The listing builds one solid part. Answer for the finished solid, in the listing's coordinates (mm). Face numbers are marked on the shaded views. Give positions to 0.01 mm unless a question says otherwise; leave off trailing zeros. Write each loop counter-clockwise with the first axis right and the second up, starting at its lowest first coordinate (ties: lowest second). Pieces come first, ordered by that corner, then holes. Notation, with made-up numbers: (-10.75, -6.75) - (24.25, -6.75) arc R5 ccw to (24.25, -1.75) - close; hole circle Ø5 at (-33.75, -27.5). An arc over 180 degrees is marked (long way). Answer as CSV lines item,"result". Start each with the question number.
(1) For a pull along Z with two mould halves and no side action, classify the marked faces 1, 2 and 3 as pulls with the +Z half, pulls with the -Z half, needs draft (parallel to the pull), parting line crosses it, or undercut.
(2) Find section C-C (x = 24.5). Write down the section's boundary in (y, z).
(3) Find section B-B (z = 14.5). Write down the section's boundary in (x, y).
(4) Straight lines are drawn through the part: probe 1 along X at (y, z) = (0.25, -11); probe 2 along Z at (x, y) = (-10.5, -2.75); probe 3 along X at (y, z) = (-13.25, 25). For each, find the intervals that lie inside material, in ascending order.
(5) Find section A-A (y = -1.75). State how many separate pieces and enclosed holes the cut face has, then the cut area to 3 significant figures.
(6) Each of these flat-tipped pins is pushed along its axis until it touches: pin 1 Ø0.8 at (y, z) = (1, -29.5) entering from +X; pin 2 Ø5 at (x, y) = (27, -3.5) entering from +Z; pin 3 Ø2.5 at (x, z) = (38.38, -39.22) entering from -Y; pin 4 Ø8 at (x, z) = (8.5, 22) entering from -Y. Where does it stop, or does it pass through?
from build123d import *

# Parameters (mm, degrees)
SKETCH1_R           = 1.375
BOSS_EXTRUDE1_DEPTH = 1.6
BOSS_EXTRUDE2_START = -17
BOSS_EXTRUDE2_DEPTH = 17
BOSS_EXTRUDE3_START = -17.6
SKETCH2_R           = 2.4
SKETCH2_R_2         = 1.375
BOSS_EXTRUDE3_DEPTH = 17.6
SKETCH3_W           = 36.288172123
SKETCH3_H           = 9.00941151
CUT_EXTRUDE1_DEPTH  = 10
SKETCH5_W           = 16.770268593
SKETCH5_H           = 4.911067329
CUT_EXTRUDE2_DEPTH  = 10
SKETCH7_W           = 55
SKETCH7_H           = 17
CUT_EXTRUDE3_DEPTH  = 10
SKETCH9_W           = 3
SKETCH9_H           = 15
CUT_EXTRUDE4_DEPTH  = 10
MOVE_FACE1_BY       = 0.4
MOVE_FACE1_2_BY     = 0.4
MOVE_FACE1_3_BY     = 0.4
MOVE_FACE1_4_BY     = 0.4
MOVE_FACE1_5_BY     = 0.4
MOVE_FACE1_6_BY     = 0.4
MOVE_FACE1_7_BY     = 0.4
MOVE_FACE1_8_BY     = 0.4
MOVE_FACE1_9_BY     = 0.4
MOVE_FACE1_10_BY    = 0.4


with BuildPart() as part:
    # Sketch1 → Boss-Extrude1 (new body)
    # profile 1 of 2: a face of its own
    with BuildSketch(Plane(origin=(0, 0, 0), x_dir=(1, 0, 0), z_dir=(0, 1, 0))):
        with BuildLine():
            Line((-11.124120265, 42.72781091), (38.875879735, 42.72781091))
            ThreePointArc((38.875879735, 42.72781091), (40.997200079, 41.849131254), (41.875879735, 39.72781091))
            Line((41.875879735, 39.72781091), (41.875879735, 36.821646567))
            Line((41.875879735, 36.821646567), (33.875879735, 36.821646567))
            Line((33.875879735, 36.821646567), (33.875879735, -16.202520779))
            Line((33.875879735, -16.202520779), (41.875879735, -16.202520779))
            Line((41.875879735, -16.202520779), (41.875879735, -39.202520779))
            ThreePointArc((41.875879735, -39.202520779), (40.997200079, -41.323841123), (38.875879735, -42.202520779))
            Line((38.875879735, -42.202520779), (-11.124120265, -42.202520779))
            ThreePointArc((-11.124120265, -42.202520779), (-13.245440608, -41.323841123), (-14.124120265, -39.202520779))
            Line((-14.124120265, -39.202520779), (-14.124120265, 39.72781091))
            ThreePointArc((-14.124120265, 39.72781091), (-13.245440608, 41.849131254), (-11.124120265, 42.72781091))
        make_face()
        with Locations(Location((-10.624120265, -18.778353433, 0), (0, 0, 270))):
            Circle(SKETCH1_R, mode=Mode.SUBTRACT)
        with Locations(Location((-10.624120265, 39.221646567, 0), (0, 0, 270))):
            Circle(SKETCH1_R, mode=Mode.SUBTRACT)
        with Locations(Location((38.375879735, 39.221646567, 0), (0, 0, 270))):
            Circle(SKETCH1_R, mode=Mode.SUBTRACT)
        with Locations(Location((38.375879735, -18.778353433, 0), (0, 0, 270))):
            Circle(SKETCH1_R, mode=Mode.SUBTRACT)
    # profile 2 of 2: a face of its own
    with BuildSketch(Plane(origin=(0, 0, 0), x_dir=(1, 0, 0), z_dir=(0, 1, 0))):
        with BuildLine():
            Line((-16.124120265, -39.202520779), (-16.124120265, 39.72781091))
            ThreePointArc((-16.124120265, 39.72781091), (-14.65965417, 43.263344816), (-11.124120265, 44.72781091))
            Line((-11.124120265, 44.72781091), (38.875879735, 44.72781091))
            ThreePointArc((38.875879735, 44.72781091), (42.411413641, 43.263344816), (43.875879735, 39.72781091))
            Line((43.875879735, 39.72781091), (43.875879735, 36.821646567))
            Line((43.875879735, 36.821646567), (41.875879735, 36.821646567))
            Line((41.875879735, 36.821646567), (41.875879735, 39.72781091))
            ThreePointArc((41.875879735, 39.72781091), (40.997200079, 41.849131254), (38.875879735, 42.72781091))
            Line((38.875879735, 42.72781091), (-11.124120265, 42.72781091))
            ThreePointArc((-11.124120265, 42.72781091), (-13.245440608, 41.849131254), (-14.124120265, 39.72781091))
            Line((-14.124120265, 39.72781091), (-14.124120265, -39.202520779))
            ThreePointArc((-14.124120265, -39.202520779), (-13.245440608, -41.323841123), (-11.124120265, -42.202520779))
            Line((-11.124120265, -42.202520779), (38.875879735, -42.202520779))
            ThreePointArc((38.875879735, -42.202520779), (40.997200079, -41.323841123), (41.875879735, -39.202520779))
            Line((41.875879735, -39.202520779), (41.875879735, -16.202520779))
            Line((41.875879735, -16.202520779), (43.875879735, -16.202520779))
            Line((43.875879735, -16.202520779), (43.875879735, -39.202520779))
            ThreePointArc((43.875879735, -39.202520779), (42.411413641, -42.738054685), (38.875879735, -44.202520779))
            Line((38.875879735, -44.202520779), (-11.124120265, -44.202520779))
            ThreePointArc((-11.124120265, -44.202520779), (-14.65965417, -42.738054685), (-16.124120265, -39.202520779))
        make_face()
    extrude(amount=BOSS_EXTRUDE1_DEPTH)

    # Sketch1<3> → Boss-Extrude2 (add)
    with BuildSketch(Plane(origin=(0, 0, 0), x_dir=(1, 0, 0), z_dir=(0, 1, 0)).offset(BOSS_EXTRUDE2_START)):
        with BuildLine():
            Line((-16.124120265, -39.202520779), (-16.124120265, 39.72781091))
            ThreePointArc((-16.124120265, 39.72781091), (-14.65965417, 43.263344816), (-11.124120265, 44.72781091))
            Line((-11.124120265, 44.72781091), (38.875879735, 44.72781091))
            ThreePointArc((38.875879735, 44.72781091), (42.411413641, 43.263344816), (43.875879735, 39.72781091))
            Line((43.875879735, 39.72781091), (43.875879735, 36.821646567))
            Line((43.875879735, 36.821646567), (41.875879735, 36.821646567))
            Line((41.875879735, 36.821646567), (41.875879735, 39.72781091))
            ThreePointArc((41.875879735, 39.72781091), (40.997200079, 41.849131254), (38.875879735, 42.72781091))
            Line((38.875879735, 42.72781091), (-11.124120265, 42.72781091))
            ThreePointArc((-11.124120265, 42.72781091), (-13.245440608, 41.849131254), (-14.124120265, 39.72781091))
            Line((-14.124120265, 39.72781091), (-14.124120265, -39.202520779))
            ThreePointArc((-14.124120265, -39.202520779), (-13.245440608, -41.323841123), (-11.124120265, -42.202520779))
            Line((-11.124120265, -42.202520779), (38.875879735, -42.202520779))
            ThreePointArc((38.875879735, -42.202520779), (40.997200079, -41.323841123), (41.875879735, -39.202520779))
            Line((41.875879735, -39.202520779), (41.875879735, -16.202520779))
            Line((41.875879735, -16.202520779), (43.875879735, -16.202520779))
            Line((43.875879735, -16.202520779), (43.875879735, -39.202520779))
            ThreePointArc((43.875879735, -39.202520779), (42.411413641, -42.738054685), (38.875879735, -44.202520779))
            Line((38.875879735, -44.202520779), (-11.124120265, -44.202520779))
            ThreePointArc((-11.124120265, -44.202520779), (-14.65965417, -42.738054685), (-16.124120265, -39.202520779))
        make_face()
    extrude(amount=BOSS_EXTRUDE2_DEPTH)

    # Sketch2 → Boss-Extrude3 (add)
    # profile 1 of 4: a face of its own
    with BuildSketch(Plane(origin=(0, 1.6, 0), x_dir=(1, 0, 0), z_dir=(0, 1, 0)).offset(BOSS_EXTRUDE3_START)):
        with Locations(Location((38.375879735, 39.221646567, 0), (0, 0, 270))):
            Circle(SKETCH2_R)
        with Locations(Location((38.375879735, 39.221646567, 0), (0, 0, 270))):
            Circle(SKETCH2_R_2, mode=Mode.SUBTRACT)
    # profile 2 of 4: a face of its own
    with BuildSketch(Plane(origin=(0, 1.6, 0), x_dir=(1, 0, 0), z_dir=(0, 1, 0)).offset(BOSS_EXTRUDE3_START)):
        with Locations(Location((38.375879735, -18.778353433, 0), (0, 0, 270))):
            Circle(SKETCH2_R)
        with Locations(Location((38.375879735, -18.778353433, 0), (0, 0, 270))):
            Circle(SKETCH2_R_2, mode=Mode.SUBTRACT)
    # profile 3 of 4: a face of its own
    with BuildSketch(Plane(origin=(0, 1.6, 0), x_dir=(1, 0, 0), z_dir=(0, 1, 0)).offset(BOSS_EXTRUDE3_START)):
        with Locations(Location((-10.624120265, -18.778353433, 0), (0, 0, 270))):
            Circle(SKETCH2_R)
        with Locations(Location((-10.624120265, -18.778353433, 0), (0, 0, 270))):
            Circle(SKETCH2_R_2, mode=Mode.SUBTRACT)
    # profile 4 of 4: a face of its own
    with BuildSketch(Plane(origin=(0, 1.6, 0), x_dir=(1, 0, 0), z_dir=(0, 1, 0)).offset(BOSS_EXTRUDE3_START)):
        with Locations(Location((-10.624120265, 39.221646567, 0), (0, 0, 270))):
            Circle(SKETCH2_R)
        with Locations(Location((-10.624120265, 39.221646567, 0), (0, 0, 270))):
            Circle(SKETCH2_R_2, mode=Mode.SUBTRACT)
    extrude(amount=BOSS_EXTRUDE3_DEPTH)

    # Sketch3 → Cut-Extrude1 (cut)
    with BuildSketch(Plane(origin=(-14.124120265, 0, 0), x_dir=(0, 0, -1), z_dir=(1, 0, 0))):
        with Locations((1.373104953, -12.495294245)):
            Rectangle(SKETCH3_W, SKETCH3_H)
    extrude(amount=-CUT_EXTRUDE1_DEPTH, mode=Mode.SUBTRACT)

    # Sketch5 → Cut-Extrude2 (cut)
    with BuildSketch(Plane.ZY.offset(16.124120265)):
        with Locations((-27.902325311, -14.544466336)):
            Rectangle(SKETCH5_W, SKETCH5_H)
    extrude(amount=-CUT_EXTRUDE2_DEPTH, mode=Mode.SUBTRACT)

    # Sketch7 → Cut-Extrude3 (cut)
    with BuildSketch(Plane.XY.offset(44.202520779)):
        with Locations((13.875879735, -8.5)):
            Rectangle(SKETCH7_W, SKETCH7_H)
    extrude(amount=-CUT_EXTRUDE3_DEPTH, mode=Mode.SUBTRACT)

    # Sketch9 → Cut-Extrude4 (cut)
    with BuildSketch(Plane(origin=(0, 1.6, 0), x_dir=(1, 0, 0), z_dir=(0, 1, 0))):
        with Locations((-4.888394882, 30.22781091)):
            Rectangle(SKETCH9_W, SKETCH9_H)
        with Locations((5.111605118, 30.22781091)):
            Rectangle(SKETCH9_W, SKETCH9_H)
        with Locations((15.111605118, 30.22781091)):
            Rectangle(SKETCH9_W, SKETCH9_H)
        with Locations((25.111605118, 30.22781091)):
            Rectangle(SKETCH9_W, SKETCH9_H)
        with Locations((5.111605118, 10.22781091)):
            Rectangle(SKETCH9_W, SKETCH9_H)
        with Locations((15.111605118, 10.22781091)):
            Rectangle(SKETCH9_W, SKETCH9_H)
        with Locations((25.111605118, 10.22781091)):
            Rectangle(SKETCH9_W, SKETCH9_H)
        with Locations((5.111605118, -9.77218909)):
            Rectangle(SKETCH9_W, SKETCH9_H)
        with Locations((15.111605118, -9.77218909)):
            Rectangle(SKETCH9_W, SKETCH9_H)
        with Locations((25.111605118, -9.77218909)):
            Rectangle(SKETCH9_W, SKETCH9_H)
        with Locations((-4.888394882, 10.22781091)):
            Rectangle(SKETCH9_W, SKETCH9_H)
        with Locations((-4.888394882, -9.77218909)):
            Rectangle(SKETCH9_W, SKETCH9_H)
    extrude(amount=-CUT_EXTRUDE4_DEPTH, mode=Mode.SUBTRACT)

    # Move Face1: a face moved inward by 0.4
    extrude(part.faces().sort_by_distance((41.375879735, -8.5, 42.196740487))[0], amount=MOVE_FACE1_BY, dir=(1, 0, 0), mode=Mode.SUBTRACT)

    # Move Face1 2: a curved face moved inward by 0.4
    add(Solid.thicken(part.faces().sort_by_distance((41.748161059, -8.5, 40.068546183))[0], -MOVE_FACE1_2_BY), mode=Mode.SUBTRACT)

    # Move Face1 3: a face moved inward by 0.4
    extrude(part.faces().sort_by_distance((41.875879735, -8.5, 27.702520779))[0], amount=MOVE_FACE1_3_BY, dir=(1, 0, 0), mode=Mode.SUBTRACT)

    # Move Face1 4: a face moved inward by 0.4
    extrude(part.faces().sort_by_distance((-13.624120265, -8.5, 42.196740487))[0], amount=MOVE_FACE1_4_BY, dir=(-1, 0, 0), mode=Mode.SUBTRACT)

    # Move Face1 5: a curved face moved inward by 0.4
    add(Solid.thicken(part.faces().sort_by_distance((-13.996401588, -8.5, 40.068546183))[0], -MOVE_FACE1_5_BY), mode=Mode.SUBTRACT)

    # Move Face1 6: a face moved inward by 0.4
    extrude(part.faces().sort_by_distance((-14.124120265, -6.565433094, 2.567801751))[0], amount=MOVE_FACE1_6_BY, dir=(-1, 0, 0), mode=Mode.SUBTRACT)

    # Move Face1 7: a curved face moved inward by 0.4
    add(Solid.thicken(part.faces().sort_by_distance((-13.245440608, -8.5, -41.849131254))[0], -MOVE_FACE1_7_BY), mode=Mode.SUBTRACT)

    # Move Face1 8: a face moved inward by 0.4
    extrude(part.faces().sort_by_distance((41.875879735, -8.5, -38.274728738))[0], amount=MOVE_FACE1_8_BY, dir=(1, 0, 0), mode=Mode.SUBTRACT)

    # Move Face1 9: a curved face moved inward by 0.4
    add(Solid.thicken(part.faces().sort_by_distance((40.997200079, -8.5, -41.849131254))[0], -MOVE_FACE1_9_BY), mode=Mode.SUBTRACT)

    # Move Face1 10: a face moved inward by 0.4
    extrude(part.faces().sort_by_distance((13.875879735, -8.5, -42.72781091))[0], amount=MOVE_FACE1_10_BY, dir=(0, 0, -1), mode=Mode.SUBTRACT)


solid = part.part
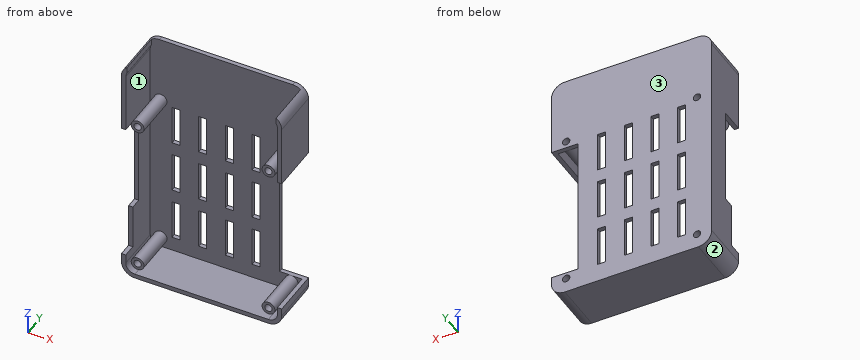
Result set:
1,face 1,"undercut"
1,face 2,"pulls with the -Z half"
1,face 3,"needs draft"
2,outline,"(-17, -44.73) - (1.6, -44.73) - (1.6, -37.73) - (0, -37.73) - (0, -43.13) - (-17, -43.13) - close; (0, -22.73) - (1.6, -22.73) - (1.6, -17.73) - (0, -17.73) - close; (0, -2.73) - (1.6, -2.73) - (1.6, 2.27) - (0, 2.27) - close; (0, 17.27) - (1.6, 17.27) - (1.6, 44.2) - (0, 44.2) - close"
3,outline,"(-16.12, -7.99) - (-14.52, -7.99) - (-14.52, 0) - (-6.39, 0) - (-6.39, 1.6) - (-16.12, 1.6) - close; (-3.39, 0) - (3.61, 0) - (3.61, 1.6) - (-3.39, 1.6) - close; (6.61, 0) - (13.61, 0) - (13.61, 1.6) - (6.61, 1.6) - close; (16.61, 0) - (23.61, 0) - (23.61, 1.6) - (16.61, 1.6) - close; (26.61, 0) - (33.88, 0) - (33.88, 1.6) - (26.61, 1.6) - close"
4,probe 1,"-16.12 to -6.39, -3.39 to 3.61, 6.61 to 13.61, 16.61 to 23.61, 26.61 to 33.88"
4,probe 2,"-44.73 to -43.13, -41.62 to -40.59, -37.85 to -36.82, 16.38 to 17.41, 20.15 to 21.18"
4,probe 3,"-16.12 to -14.52, 42.28 to 43.88"
5,separate pieces,"6"
5,enclosed holes,"4"
5,area,"328 mm^2"
6,pin 1,"x = 33.88"
6,pin 2,"z = -43.13"
6,pin 3,"through"
6,pin 4,"y = 0"
